Here's the drawing with two shaded views (mm, measured from the low corner). I have some questions. Coordinates: 2 decimals unless noted, no trailing zeros. Write each loop counter-clockwise with the first axis right and the second up, starting at its lowest first coordinate (ties: lowest second). Pieces come first, ordered by that corner, then holes.
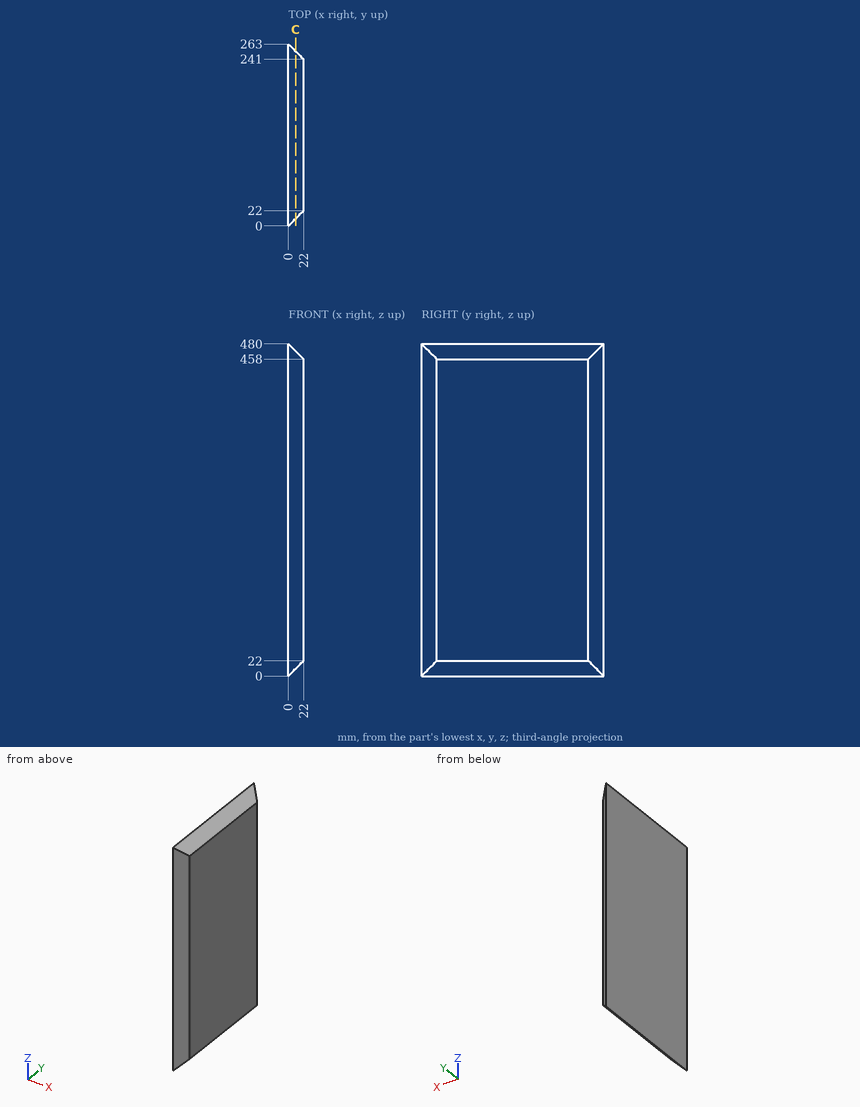
1. Please list where these lines run through material, in increasing order: line 1 along Y through (x, z) = (16.25, 282.5); line 2 along Y through (x, z) = (20.5, 279.5); line 3 along Z through (x, y) = (19, 49.5).
Verdict:
line 1: y = 16.25 to 246.75
line 2: y = 20.5 to 242.5
line 3: z = 19 to 461
2. I want a section at C-C on x = 10.5. Please give me the cut outline in (y, z).
Verdict:
outline: (10.5, 10.5) - (252.5, 10.5) - (252.5, 469.5) - (10.5, 469.5) - close
3. For pin 1 (8 mm diameter, centred on x = 7, z = 356, fed in from -Y); pin 2 (6 mm diameter, centred on x = 17, z = 269.5, fed in from -Y); pin 3 (3 mm diameter, centred on x = 19, z = 178, fed in from +Y), each with a flat end and sliding along its axis, tell me the tip position at first contact or that it passes through.
Verdict:
pin 1: stops at y = 3
pin 2: stops at y = 14
pin 3: stops at y = 245.5
